Verification items for the finished model (mm, model axes). A direction names the side the tool comes from. Coordinates: 2 decimals unless noted, no trailing zeros. Order: outer loops, then holes, each group sorted by start corner. A loop starts at its lowest first (then second) coordinate and runs counter-clockwise, first axis right, second up. Notation, with made-up numbers: M 56.25,-36 L 64.25,-36 A14 ccw 64.25,-30 Z; hole C 31,58 d1. An arc over 180 degrees is marked long. Answer as a JSON object with one key per item and string values. Group by question number.
(1) Material ranges on line 1 (Z direction, x = -3, y = -61.5); line 2 (Y direction, x = -0.5, z = 112); line 3 (X direction, y = 2, z = 24.5), recorded low to high.
(2) Cross-section at B-B (y = 0). Enter the section's corners in (x, z), plus the area to 3 significant figures.
(3) Mould release check, pull along X, two halves, no side actions. Record for faces 1 (the face through (-33.62, 51.396, 12.021)), 2 (the face through (11.81, 3.72, 98.26)), 3 (the face through (-1, -15, 24.384)), 4 (the face through (-91.44, 0, 155)): released by +X, released by -X, zero draft, split by the parting line, or undercut.
(4) Gauge pin test, flat ends, axial feed: pin 1 Ø3 at (y, z) = (0.5, 154.5) entering from +X; pin 2 Ø3 at (x, y) = (48, 40) entering from +Z; pin 3 Ø3 at (x, z) = (-12.5, 152.5) entering from -Y. Record the tip position at first contact, or that the pin passes through.
(5) Access from +Z, -Z, +X, -X, +Y, -Y to the whole of each face (thin tool, end or side, straight path). Record for faces 5 (the face through (-1, 1, 0)), 6 (the face through (0, 0, 174.244)), 7 (the face through (-50.78, -1.13, 149.44)), 8 (the face through (12.7, 0, 155)), 9 (the face through (12.141, -3.836, 158.039)).
(6) Cross-section at C-C (x = 0). Enter the section's corners in (y, z), plus the area to 3 significant figures.
(7) Cross-section at A-A (x = -32.5). Enter the section's corners in (y, z), plus the area to 3 significant figures.
(8) Cross-section at D-D (z = 72.5). Enter the section's corners in (x, y).
from build123d import *

# Parameters (mm, degrees)
F0_R     = 12.381892
F1_DEPTH = 174.244
F3_R     = 5.204488
F4_DEPTH = 104.14
F5_R     = 73.405341
F6_DEPTH = 24.384
F7_R     = 10.235871
F8_DEPTH = 25.4


with BuildPart() as f1:
    # F0 (on Top) → F1 (new body)
    with BuildSketch(Plane.XY):
        Circle(F0_R)
    extrude(amount=F1_DEPTH)

    # F3 (on offset) → F4 (join)
    with BuildSketch(Plane.YZ.offset(12.7)):
        with Locations((0, 154.521525)):
            Circle(F3_R)
    extrude(amount=-F4_DEPTH)

    # F5 (on Top) → F6 (join)
    with BuildSketch(Plane.XY):
        Circle(F5_R)
    extrude(amount=F6_DEPTH)

    # F7 (on Top) → F8 (cut)
    with BuildSketch(Plane.XY):
        with Locations((-26.076123, 44.477817)):
            Circle(F7_R)
    extrude(amount=F8_DEPTH, mode=Mode.SUBTRACT)


solid = f1.part
Taken from the geometry:
{
 "1": {"line 1": "z = 0 to 24.38", "line 2": "y = -12.37 to 12.37", "line 3": "x = -12.22 to 12.22"},
 "2": {"outline": "M -91.44,149.32 L -12.38,149.32 L -12.38,24.38 L -73.41,24.38 L -73.41,0 L 73.41,0 L 73.41,24.38 L 12.38,24.38 L 12.38,149.32 L 12.7,149.32 L 12.7,159.73 L 12.38,159.73 L 12.38,174.24 L -12.38,174.24 L -12.38,159.73 L -91.44,159.73 Z", "area": "8,120 mm²"},
 "3": {"face 1": "undercut", "face 2": "split by the parting line", "face 3": "zero draft", "face 4": "released by -X"},
 "4": {"pin 1": "stops at x = 12.7", "pin 2": "stops at z = 24.38", "pin 3": "stops at y = -5.68"},
 "5": {"face 5": "-Z, +X, -X, +Y, -Y", "face 6": "+Z, +X, -X, +Y, -Y", "face 7": "-X", "face 8": "+Z, +X, +Y, -Y", "face 9": "+X"},
 "6": {"outline": "M -73.41,0 L 73.41,0 L 73.41,24.38 L 12.38,24.38 L 12.38,174.24 L -12.38,174.24 L -12.38,24.38 L -73.41,24.38 Z", "area": "7,290 mm²"},
 "7": {"outline": "M -65.82,0 L 36.51,0 L 36.51,24.38 L -65.82,24.38 Z; C 0,154.52 d10.41; M 52.45,0 L 65.82,0 L 65.82,24.38 L 52.45,24.38 Z", "area": "2,910 mm²"},
 "8": {"outline": "C 0,0 d24.76"}
}
